Geometry check sheet. Reference: the model listing, model coordinates, mm. A direction names the side the tool comes from. Round coordinates to 2 decimals unless told otherwise and drop trailing zeros. Write each loop counter-clockwise with the first axis right and the second up, starting at its lowest first coordinate (ties: lowest second). Pieces come first, ordered by that corner, then holes. Notation, with made-up numbers: (0, 21) - (35, 21) arc R7 ccw to (35, 27) - close; hole circle Ø2 at (-5, 78.5). An arc over 180 degrees is marked (long way). Return JSON: item names as keys, results as strings.
```python
from build123d import *

# Parameters (mm, degrees)
SKETCH1_W           = 35
SKETCH1_H           = 15
SKETCH1_R           = 1
SKETCH1_W_2         = 23.5
SKETCH1_H_2         = 13
BOSS_EXTRUDE1_DEPTH = 2
SKETCH2_W           = 2
SKETCH2_H           = 5
CUT_EXTRUDE1_DEPTH  = 2


with BuildPart() as part:
    # Sketch1 → Boss-Extrude1 (new body)
    with BuildSketch(Plane(origin=(0, 0, 0), x_dir=(1, 0, 0), z_dir=(0, 1, 0))):
        Rectangle(SKETCH1_W, SKETCH1_H)
        with Locations(Location((-13.5, 0, 0), (0, 0, 270))):
            Circle(SKETCH1_R, mode=Mode.SUBTRACT)
        with Locations(Location((13.5, 0, 0), (0, 0, 90))):
            Circle(SKETCH1_R, mode=Mode.SUBTRACT)
        Rectangle(SKETCH1_W_2, SKETCH1_H_2, mode=Mode.SUBTRACT)
    extrude(amount=BOSS_EXTRUDE1_DEPTH)

    # Sketch2 → Cut-Extrude1 (cut)
    with BuildSketch(Plane(origin=(0, 2, 0), x_dir=(1, 0, 0), z_dir=(0, 1, 0))):
        with Locations((16.5, 5)):
            Rectangle(SKETCH2_W, SKETCH2_H)
        with Locations((16.5, -5)):
            Rectangle(SKETCH2_W, SKETCH2_H)
        with Locations((-16.5, -5)):
            Rectangle(SKETCH2_W, SKETCH2_H)
        with Locations((-16.5, 5)):
            Rectangle(SKETCH2_W, SKETCH2_H)
    extrude(amount=-CUT_EXTRUDE1_DEPTH, mode=Mode.SUBTRACT)


solid = part.part
```
(1) Gauge pin test, flat ends, axial feed: pin 1 (1 mm diameter, centred on y = 1, z = -5, fed in from +X); pin 2 (0.6 mm diameter, centred on x = 16.5, y = 1, fed in from +Z); pin 3 (0.6 mm diameter, centred on y = 0.5, z = 4, fed in from -X). Record the tip position at first contact, or that the pin passes through.
Response values:
{"pin 1": "stops at x = 15.5", "pin 2": "stops at z = 2.5", "pin 3": "stops at x = -15.5"}
(2) Access from +Z, -Z, +X, -X, +Y, -Y to the whole of each face (thin tool, end or side, straight path). Record for faces 1 (the face through (-11.75, 1, 0)), 2 (the face through (16, 1, 2.5)), 3 (the face through (-15.5, 1, -5)), 4 (the face through (-15.5, 1, 5)), 5 (the face through (16, 1, -2.5)).
Response values:
{"face 1": "+Y, -Y", "face 2": "+Z, +X, +Y, -Y", "face 3": "-Z, -X, +Y, -Y", "face 4": "+Z, -X, +Y, -Y", "face 5": "-Z, +X, +Y, -Y"}
(3) Material ranges on line 1 along X through (y, z) = (0.4, 0); line 2 along Z through (x, y) = (8.5, 0.1); line 3 along X through (y, z) = (0.25, 2), recorded low to high. Write a range as [from, to].
Response values:
{"line 1": "x = [-17.5, -14.5], [-12.5, -11.75], [11.75, 12.5], [14.5, 17.5]", "line 2": "z = [-7.5, -6.5], [6.5, 7.5]", "line 3": "x = [-17.5, -11.75], [11.75, 17.5]"}
(4) Section check A-A, the plane z = -4.75. Enter the section's corners in (x, y), plus the area to 3 significant figures.
Response values:
{"outline": "(-15.5, 0) - (-11.75, 0) - (-11.75, 2) - (-15.5, 2) - close; (11.75, 0) - (15.5, 0) - (15.5, 2) - (11.75, 2) - close", "area": "15.0 mm^2"}
(5) Section check B-B, the plane x = -2. Enter the section's corners in (y, z), plus the area to 3 significant figures.
Response values:
{"outline": "(0, -7.5) - (2, -7.5) - (2, -6.5) - (0, -6.5) - close; (0, 6.5) - (2, 6.5) - (2, 7.5) - (0, 7.5) - close", "area": "4.00 mm^2"}
(6) Section check D-D, the plane z = 0. Enter the section's corners in (x, y), plus the area to 3 significant figures.
Response values:
{"outline": "(-17.5, 0) - (-14.5, 0) - (-14.5, 2) - (-17.5, 2) - close; (-12.5, 0) - (-11.75, 0) - (-11.75, 2) - (-12.5, 2) - close; (11.75, 0) - (12.5, 0) - (12.5, 2) - (11.75, 2) - close; (14.5, 0) - (17.5, 0) - (17.5, 2) - (14.5, 2) - close", "area": "15.0 mm^2"}
(7) Release check for a two-part mould opening along Z. For faces 6 (the face through (17.5, 1, 0)), 7 (the face through (-17, 1, -2.5)), 8 (the face through (-14.476, 0.986, -0.217)) record: pulls with the +Z half, pulls with the -Z half, needs draft (parallel to the pull), parting line crosses it, or undercut.
Response values:
{"face 6": "needs draft", "face 7": "pulls with the -Z half", "face 8": "undercut"}
(8) Section check C-C, the plane y = 0.75. Enter the section's corners in (x, z), plus the area to 3 significant figures.
Response values:
{"outline": "(-17.5, -2.5) - (-15.5, -2.5) - (-15.5, -7.5) - (15.5, -7.5) - (15.5, -2.5) - (17.5, -2.5) - (17.5, 2.5) - (15.5, 2.5) - (15.5, 7.5) - (-15.5, 7.5) - (-15.5, 2.5) - (-17.5, 2.5) - close; hole circle Ø2 at (-13.5, 0); hole (-11.75, -6.5) - (11.75, -6.5) - (11.75, 6.5) - (-11.75, 6.5) - close; hole circle Ø2 at (13.5, 0)", "area": "173 mm^2"}
